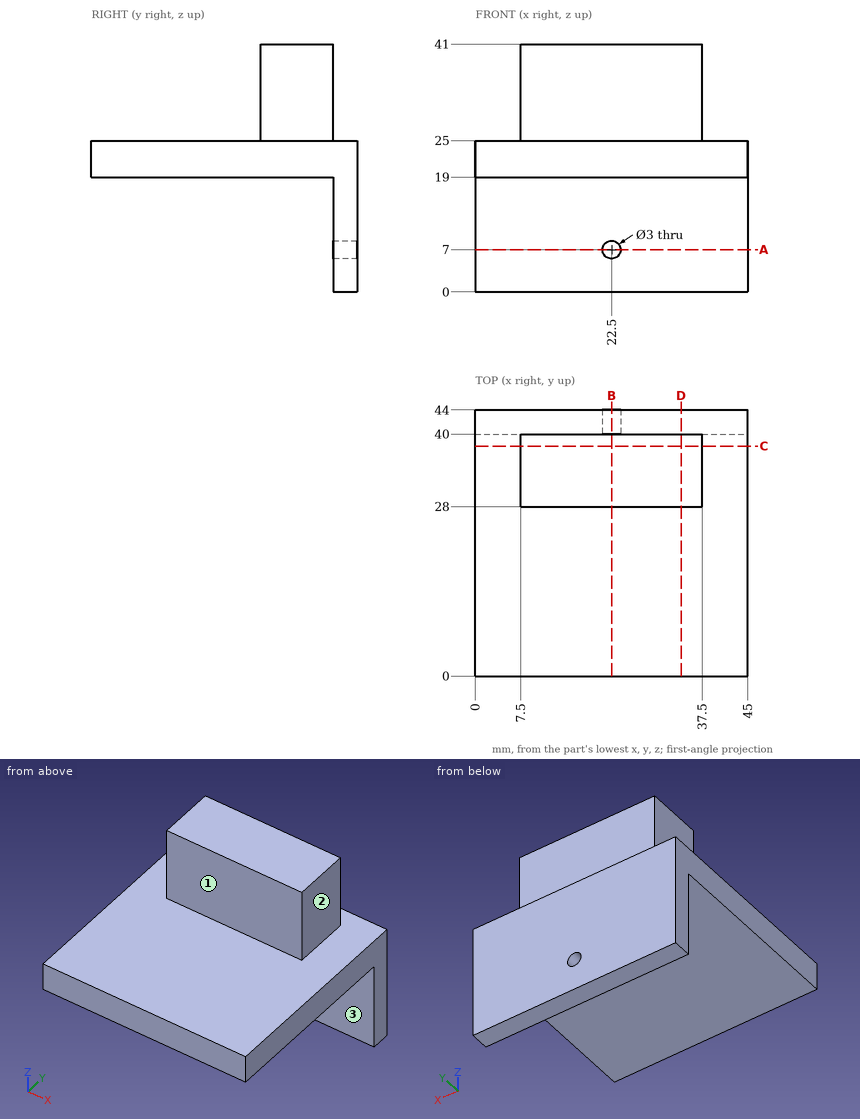
Source: three-view drawing plus pictorial views. Frame: mm from the lowest corner of the part. A direction names the side the tool comes from. Round coordinates to 2 decimals unless told otherwise and drop trailing zeros. Loops run counter-clockwise (first coordinate to the right, second up) from the corner with the lowest first, then second, coordinate; pieces in that order, holes last.
Q1. Section D-D, the plane x = 34. Return loops of the section in (y, z).
Q2. Section B-B, the plane x = 22.5. Return loops of the section in (y, z).
Q3. Ray query, line 1 (X direction, y = 43, z = 7); line 2 (X direction, y = 33, z = 37.5); line 3 (Y direction, x = 36, z = 11). Return the intervals inside material, ascending.
Q4. First-contact query: P1, Ø1, axis at x = 15.5, z = 18, coming from the -Y side; P2, Ø13, axis at x = 18.5, z = 34.5, coming from the -Y side; P3, Ø6, axis at x = 17.5, y = 9, coming from the -Z side; P4, Ø2.5, axis at x = 22.5, z = 7, coming from the +Y side. Flat tips, straight axial feed; report the tip coordinate or a pass-through.
Q5. Section C-C, the plane y = 38. Return loops of the section in (x, z).
Q6. Access query for the marked faces 1, 2 and 3. Directions: +Z, -Z, +X, -X, +Y, -Y. A direction counts if a zero-diameter tool reaches every point of the face in a straight line with its end or side. Return the directions, or none.
Q7. Section A-A, the plane z = 7. Return loops of the section in (x, y).
Solutions:
1. outline: (0, 19) - (40, 19) - (40, 0) - (44, 0) - (44, 25) - (40, 25) - (40, 41) - (28, 41) - (28, 25) - (0, 25) - close
2. outline: (0, 19) - (40, 19) - (40, 8.5) - (44, 8.5) - (44, 25) - (40, 25) - (40, 41) - (28, 41) - (28, 25) - (0, 25) - close; (40, 0) - (44, 0) - (44, 5.5) - (40, 5.5) - close
3. line 1: x = 0 to 21, 24 to 45
3. line 2: x = 7.5 to 37.5
3. line 3: y = 40 to 44
4. P1: stops at y = 40
4. P2: stops at y = 28
4. P3: stops at z = 19
4. P4: passes through
5. outline: (0, 19) - (45, 19) - (45, 25) - (37.5, 25) - (37.5, 41) - (7.5, 41) - (7.5, 25) - (0, 25) - close
6. face 1: +Z, +X, -X, -Y
6. face 2: +Z, +X, +Y, -Y
6. face 3: -Z, +X, -X, -Y
7. outline: (0, 40) - (21, 40) - (21, 44) - (0, 44) - close; (24, 40) - (45, 40) - (45, 44) - (24, 44) - close
